For this review, take the finished solid that the model builds, in its own axes (mm). Face numbers are marked on the shaded views. A direction names the side the tool comes from. Give positions to 0.01 mm unless a question says otherwise; leave off trailing zeros. Loops run counter-clockwise (first coordinate to the right, second up) from the corner with the lowest first, then second, coordinate; pieces in that order, holes last. Notation, with made-up numbers: (1.25, 71) - (45.25, 71) arc R14 ccw to (45.25, 97) - close; hole circle Ø8 at (33, -21). An arc over 180 degrees is marked (long way). Answer as CSV lines item,"result".
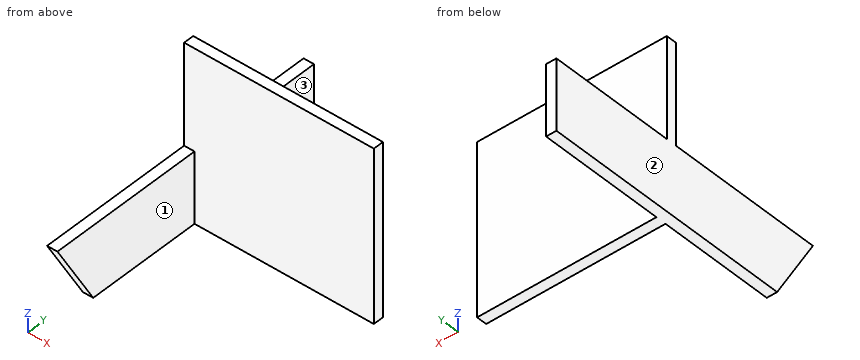
from build123d import *

# Parameters (mm, degrees)
PAD_DEPTH         = 2
SKETCH001_W       = 2
SKETCH001_H       = 33.12
PAD001_DEPTH      = 34.6
PAD001_DEPTH_BACK = 2


with BuildPart() as part:
    # Sketch → Pad (new body)
    with BuildSketch(Plane.YZ):
        Polygon((-23.355, 0), (25.355, 0), (25.355, 13.665881), (-31.245, 13.665881), align=None)
    extrude(amount=PAD_DEPTH)

    # Sketch001 (on Face6 of Pad) → Pad001 (join, two sides)
    with BuildSketch(Plane.YZ.offset(2)) as pad001_sk:
        with Locations((0, 16.56)):
            Rectangle(SKETCH001_W, SKETCH001_H)
    extrude(amount=PAD001_DEPTH)
    extrude(pad001_sk.sketch, amount=-PAD001_DEPTH_BACK)


solid = part.part
1) Insertion check: P1, Ø1, axis at x = 12, z = 29, coming from the -Y side; P2, Ø1.6, axis at x = 0.5, y = 13.5, coming from the +Z side; P3, Ø16.5, axis at x = 21, z = 17, coming from the +Y side. Each pin has a flat end and moves straight along its axis. Give the tip position at first contact, or say it passes through.
From the geometry:
P1,"stops at y = -1"
P2,"stops at z = 13.67"
P3,"stops at y = 1"
2) Consider section C-C on y = -27. Write out the cut boundary in (x, z), and give its area (3 significant figures).
From the geometry:
outline,"(0, 6.31) - (2, 6.31) - (2, 13.67) - (0, 13.67) - close"
area,"14.7 mm^2"
3) Consider section A-A on z = 11.5. Write out the cut boundary in (x, y) (3 decimals).
From the geometry:
outline,"(0, -29.995) - (2, -29.995) - (2, -1) - (36.6, -1) - (36.6, 1) - (2, 1) - (2, 25.355) - (0, 25.355) - close"
4) Consider section B-B on x = 32.5. Write out the cut boundary in (y, z), and give its area (3 significant figures).
From the geometry:
outline,"(-1, 0) - (1, 0) - (1, 33.12) - (-1, 33.12) - close"
area,"66.2 mm^2"
5) Machinability: for the marked faces 1, 2 and 3, which of the approach directions +Z, -Z, +X, -X, +Y, -Y give a long, thin tool a straight path to every point of the face, cutting with its end or side? Answer none if there is none.
From the geometry:
face 1,"+Z, -Z, +X, -Y"
face 2,"+Z, -Z, -X, +Y, -Y"
face 3,"+Z, -Z, +X, +Y"
6) Wall thickness on line 1 (Y direction, x = 33.5, z = 5); line 2 (X direction, y = 13, z = 4): over which ranges is each line inside the solid? List them lowest first. Write a range as from..to.
From the geometry:
line 1,"y = -1..1"
line 2,"x = 0..2"
7) Consider section D-D on z = 4.5. Write out the cut boundary in (x, y) (3 decimals).
From the geometry:
outline,"(0, -25.953) - (2, -25.953) - (2, -1) - (36.6, -1) - (36.6, 1) - (2, 1) - (2, 25.355) - (0, 25.355) - close"
